Could you check a few things on this model? Use its own coordinates, in mm. Face numbers are marked on the shaded views. Give positions to 0.01 mm unless a question says otherwise; leave off trailing zeros. Loops run counter-clockwise (first coordinate to the right, second up) from the corner with the lowest first, then second, coordinate; pieces in that order, holes last. Notation, with made-up numbers: (84.5, -38.75) - (137.5, -38.75) arc R15 ccw to (137.5, -16.75) - close; hole circle Ø11 at (77.25, 55). An arc over 180 degrees is marked (long way). One line per item, written item: value. Start each with the question number.
Q1. I want a section at A-A (y = 1). Please give me the cut outline in (x, z), then the cut area to 3 significant figures.
Q2. I'm going to push flat-ended pins straight in: P1, Ø11.5, axis at x = 0, z = -1, coming from the +Y side; P2, Ø5.5, axis at x = -4, z = 12, coming from the +Y side; P3, Ø8, axis at x = -7, z = 10, coming from the -Y side; P4, Ø0.8, axis at x = -1.5, y = 11, coming from the +Z side (3 decimals). Where does each tip first touch, or does it pass through?
Q3. If we mould it in two halves opening along Z, with no side actions, what happens to the marked faces 1, 2, 3 and 4? For each: released by +Z, released by -Z, zero draft, split by the parting line, or undercut.
Q4. I want a section at C-C (x = 7). Please give me the cut outline in (y, z), then the cut area to 3 significant figures.
Q5. If I drill on line 1 (X direction, y = 8, z = 0); line 2 (X direction, y = 6.5, z = 12.5); line 3 (Z direction, x = 5.5, y = 7.5), over which ranges is the centre line in solid material (lowest first)? Write a range as from..to.
Q6. I want a section at B-B (z = 12.5). Please give me the cut outline in (x, y).
Q7. I want a section at D-D (y = 5.5). Please give me the cut outline in (x, z).
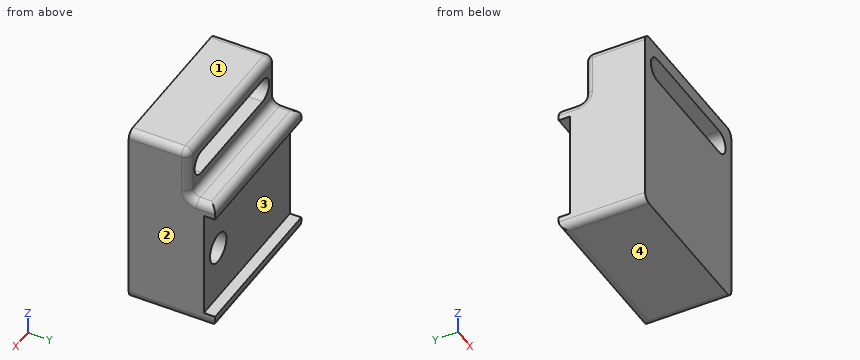
```python
from build123d import *

# Parameters (mm, degrees)
SKETCH1_W           = 21
SKETCH1_H           = 14.6
BOSS_EXTRUDE1_DEPTH = 10
SKETCH1_3_W         = 21
SKETCH1_3_H         = 1.7
BOSS_EXTRUDE2_DEPTH = 11.5
SKETCH3_W           = 21
SKETCH3_H           = 7
BOSS_EXTRUDE4_DEPTH = 8
FILLET1_R           = 1
CUT_EXTRUDE1_DEPTH  = 21.742468513
SKETCH5_R           = 2
CUT_EXTRUDE2_DEPTH  = 6.8


with BuildPart() as part:
    # Sketch1 → Boss-Extrude1 (new body)
    with BuildSketch(Plane(origin=(0, 0, 0), x_dir=(1, 0, 0), z_dir=(0, 1, 0))):
        Rectangle(SKETCH1_W, SKETCH1_H)
    extrude(amount=BOSS_EXTRUDE1_DEPTH)

    # Sketch1_3 → Boss-Extrude2 (add)
    with BuildSketch(Plane(origin=(0, 0, 0), x_dir=(1, 0, 0), z_dir=(0, 1, 0))):
        with Locations((0, -8.15)):
            Rectangle(SKETCH1_3_W, SKETCH1_3_H)
        with Locations((0, 8.15)):
            Rectangle(SKETCH1_3_W, SKETCH1_3_H)
    extrude(amount=BOSS_EXTRUDE2_DEPTH)

    # Sketch3 → Boss-Extrude4 (add)
    with BuildSketch(Plane(origin=(0, 0, 0), x_dir=(1, 0, 0), z_dir=(0, 1, 0))):
        with Locations((0, -12.5)):
            Rectangle(SKETCH3_W, SKETCH3_H)
    extrude(amount=BOSS_EXTRUDE4_DEPTH)

    # Fillet1
    fillet1_edges = [part.edges().sort_by_distance(p)[0] for p in [
        (10.5, 9.75, 9),
        (-10.5, 9.75, 9),
        (0, 11.5, 9),
        (0, 11.5, -9),
        (10.5, 5.75, -9),
        (-10.5, 5.75, -9),
        (-10.5, 4, 16),
        (10.5, 4, 16),
        (-10.5, 8, 12.5),
        (0, 8, 16),
        (10.5, 8, 12.5),
        (0, 8, 9),
    ]]
    fillet(fillet1_edges, radius=FILLET1_R)

    # Sketch4 → Cut-Extrude1 (cut, through all)
    with BuildSketch(Plane(origin=(0, 8, 0), x_dir=(1, 0, 0), z_dir=(0, 1, 0))):
        with BuildLine():
            Line((-7.5, -10.9), (7.5, -10.9))
            ThreePointArc((7.5, -10.9), (9.1, -12.5), (7.5, -14.1))
            Line((7.5, -14.1), (-7.5, -14.1))
            ThreePointArc((-7.5, -14.1), (-9.1, -12.5), (-7.5, -10.9))
        make_face()
    extrude(amount=-CUT_EXTRUDE1_DEPTH, mode=Mode.SUBTRACT)

    # Sketch5 → Cut-Extrude2 (cut)
    with BuildSketch(Plane(origin=(0, 10, 0), x_dir=(1, 0, 0), z_dir=(0, 1, 0))):
        with Locations(Location((7, 0, 0), (0, 0, 270))):
            Circle(SKETCH5_R)
    extrude(amount=-CUT_EXTRUDE2_DEPTH, mode=Mode.SUBTRACT)


solid = part.part
```
Worked answers:
1. outline: (-10.5, -8) arc R1 ccw to (-9.5, -9) - (9.5, -9) arc R1 ccw to (10.5, -8) - (10.5, 15) arc R1 ccw to (9.5, 16) - (-9.5, 16) arc R1 ccw to (-10.5, 15) - close; hole (-7.5, 10.9) - (7.5, 10.9) arc R1.6 ccw to (7.5, 14.1) - (-7.5, 14.1) arc R1.6 ccw to start
1. area: 468 mm²
2. P1: stops at y = 10
2. P2: stops at y = 8.34
2. P3: stops at y = 0
2. P4: stops at z = 8.995
3. face 1: released by +Z
3. face 2: zero draft
3. face 3: undercut
3. face 4: released by -Z
4. outline: (0, -9) - (10.5, -9) arc R1 ccw to (11.5, -8) - (11.5, -7.3) - (10, -7.3) - (10, -2) - (3.2, -2) - (3.2, 2) - (10, 2) - (10, 7.3) - (11.5, 7.3) - (11.5, 8) arc R1 ccw to (10.5, 9) - (9, 9) arc R1 cw to (8, 10) - (8, 10.9) - (0, 10.9) - close; (0, 14.1) - (8, 14.1) - (8, 15) arc R1 ccw to (7, 16) - (0, 16) - close
4. area: 188 mm²
5. line 1: x = -10.5..5, 9..10.5
5. line 2: x = -10.5..-9.1, 9.1..10.5
5. line 3: z = -9..-1.32, 1.32..10.9, 14.1..15.87
6. outline: (-10.5, 0) - (-9.1, 0) - (-9.1, 8) - (-9.5, 8) arc R1 ccw to (-10.5, 7) - close; (9.1, 0) - (10.5, 0) - (10.5, 7) arc R1 ccw to (9.5, 8) - (9.1, 8) - close
7. outline: (-10.5, -8) arc R1 ccw to (-9.5, -9) - (9.5, -9) arc R1 ccw to (10.5, -8) - (10.5, 15) arc R1 ccw to (9.5, 16) - (-9.5, 16) arc R1 ccw to (-10.5, 15) - close; hole (-7.5, 10.9) - (7.5, 10.9) arc R1.6 ccw to (7.5, 14.1) - (-7.5, 14.1) arc R1.6 ccw to start; hole circle Ø4 at (7, 0)
